Verification items for the finished model (mm, model axes). A direction names the side the tool comes from. Give positions to 0.01 mm unless a question says otherwise; leave off trailing zeros. Order: outer loops, then holes, each group sorted by start corner. A loop starts at its lowest first (then second) coordinate and runs counter-clockwise, first axis right, second up. Notation, with made-up numbers: M -26,40.25 L 31,40.25 A24 cw 31,72.25 Z; hole C 31.5,69 d4. An arc over 180 degrees is marked long. Answer as a JSON object with one key per item and string values.
```python
from build123d import *

# Parameters (mm, degrees)
BOSS_EXTRUDE1_DEPTH = 3.25
SKETCH2_W           = 60
SKETCH2_H           = 10
CUT_EXTRUDE1_DEPTH  = 4
CHAMFER1_SIZE       = 5
FILLET1_R           = 1


with BuildPart() as part:
    # Sketch1 → Boss-Extrude1 (new, symmetric)
    with BuildSketch(Plane(origin=(0, 0, 0), x_dir=(1, 0, 0), z_dir=(0, 1, 0))):
        Polygon((-50, 10), (-30, -10), (30, -10), (50, 10), align=None)
    extrude(amount=BOSS_EXTRUDE1_DEPTH, both=True)

    # Sketch2 → Cut-Extrude1 (cut)
    with BuildSketch(Plane.XZ.offset(3.25)):
        with Locations((0, -5)):
            Rectangle(SKETCH2_W, SKETCH2_H)
    extrude(amount=-CUT_EXTRUDE1_DEPTH, mode=Mode.SUBTRACT)

    # Sketch3 → Cut-Revolve1 (revolve, cut)
    with BuildSketch(Plane(origin=(-30, 0, 0), x_dir=(0, 0, -1), z_dir=(1, 0, 0))):
        with BuildLine():
            Line((5, -0.25), (5, -2.25))
            ThreePointArc((5, -2.25), (6, -1.25), (5, -0.25))
        make_face()
    revolve(axis=Axis((-30, -0.25, -5), (0, -1, 0)), mode=Mode.SUBTRACT)

    # Sketch4 → Cut-Revolve2 (revolve, cut)
    with BuildSketch(Plane.ZY.offset(-30)):
        with BuildLine():
            Line((-5, -0.25), (-5, -2.25))
            ThreePointArc((-5, -2.25), (-6, -1.25), (-5, -0.25))
        make_face()
    revolve(axis=Axis((30, 0.75, -5), (0, -1, 0)), mode=Mode.SUBTRACT)

    # Chamfer1
    chamfer1_edges = [part.edges().sort_by_distance(p)[0] for p in [
        (0, 3.25, 10),
    ]]
    chamfer(chamfer1_edges, length=CHAMFER1_SIZE)

    # Fillet1
    fillet1_edges = [part.edges().sort_by_distance(p)[0] for p in [
        (-30, -1.25, -10),
        (-30, -1.25, 0),
        (30, -1.25, 0),
        (30, -1.25, -10),
        (-50, 0, -10),
        (50, 0, -10),
    ]]
    fillet(fillet1_edges, radius=FILLET1_R)


solid = part.part
```
Q1. Tool access check on faces 1 (the face through (39, 0, 1)), 2 (the face through (-30, -2, -6)). Record the directions out of +Z, -Z, +X, -X, +Y, -Y that give a thin tool (end or side, any length) a straight path to the whole face; none if there is none.
Resolved:
{"face 1": "+Z, +X, +Y, -Y", "face 2": "-Z, -Y"}
Q2. Release check for a two-part mould opening along X. For faces 3 (the face through (1, 1, -10)), 4 (the face through (0, 0.75, -5)), 5 (the face through (-39, 0, 1)), 6 (the face through (30, -2, -6)) record: +X half, -X half, draft (parallel to the pull), parting line (faces both ways), or undercut.
Resolved:
{"face 3": "draft", "face 4": "undercut", "face 5": "-X half", "face 6": "undercut"}
Q3. Section check A-A on x = 11.5. Record the cut outline in (y, z), then the cut area to 3 significant figures.
Resolved:
{"outline": "M -3.25,0 L 0.75,0 L 0.75,-10 L 3.25,-10 L 3.25,5 L -1.75,10 L -3.25,10 Z", "area": "77.5 mm²"}
Q4. Gauge pin test, flat ends, axial feed: pin 1 Ø1.2 at (x, y) = (-12, -1) entering from -Z; pin 2 Ø3 at (y, z) = (-1, -6) entering from -X; pin 3 Ø1.2 at (y, z) = (-1.5, -5.5) entering from +X. Record the tip position at first contact, or that the pin passes through.
Resolved:
{"pin 1": "stops at z = 0", "pin 2": "stops at x = -47.5", "pin 3": "stops at x = 46.1"}
Q5. Material ranges on L1, parallel to Y at x = 5.5, z = 8.25; L2, parallel to Z at x = 24, y = -2; L3, parallel to Y at x = -8.5, z = -0.25, recorded low to high.
Resolved:
{"L1": "y = -3.25 to 0", "L2": "z = 0 to 10", "L3": "y = 0.75 to 3.25"}
Q6. Section check C-C on y = 2. Record the cut outline in (x, z).
Resolved:
{"outline": "M -48.29,-8.29 A1 ccw -47.59,-10 L 47.59,-10 A1 ccw 48.29,-8.29 L 33.75,6.25 L -33.75,6.25 Z"}
Q7. Section check D-D on z = 6.5. Record the cut outline in (x, y).
Resolved:
{"outline": "M -33.5,-3.25 L 33.5,-3.25 L 33.5,1.75 L -33.5,1.75 Z"}
Q8. Section check B-B on z = -2.75. Record the cut outline in (x, y).
Resolved:
{"outline": "M -42.75,-3.25 L -30,-3.25 L -30,0.75 L 30,0.75 L 30,-3.25 L 42.75,-3.25 L 42.75,3.25 L -42.75,3.25 Z"}
